Check sheet for the drawn part. Datum: minimum x, y, z corner. Units: mm. A direction names the side the tool comes from. Coordinates: 2 decimals unless noted, no trailing zeros. Write each loop counter-clockwise with the first axis right and the second up, starting at its lowest first coordinate (ties: lowest second). Pieces come first, ordered by that corner, then holes. Notation, with made-up numbers: (-10.5, 33.5) -> (37.5, 33.5) arc R37 ccw to (37.5, 72.5) -> close; hole circle Ø5 at (84, -33.5). An arc over 180 degrees is marked (long way). Answer in a Markdown table with one row per item. Add a question column.
1. Depth check by flat-ended pin: P1, Ø4, axis at x = 11.5, y = 16.5, coming from the -Z side; P2, Ø12, axis at x = 14, z = 17.5, coming from the -Y side; P3, Ø1.6, axis at x = 11.5, y = 17.5, coming from the -Z side. Enter the tip coordinate at first touch or a pass-through.
2. Set-up check for the marked faces 1 and 2: record each of +Z, -Z, +X, -X, +Y, -Y from which the full face is reachable in a straight line by a thin tool's end or side.
3. Mould release check, pull along X, two halves, no side actions. Record for the marked faces 3 and 4: pulls with the +X half, pulls with the -X half, needs draft (parallel to the pull), parting line crosses it, or undercut.
4. Cross-section at C-C on z = 10.5. Record the cut outline in (x, y), and give its area (3 significant figures).
5. Cross-section at B-B on z = 17.5. Record the cut outline in (x, y), and give its area (3 significant figures).
6. Cross-section at A-A on x = 11.4. Record the cut outline in (y, z), and give its area (3 significant figures).
7. Scan lines: L1, parallel to Z at x = 7, y = 11.75; L2, parallel to Y at x = 17.25, z = 2.75; L3, parallel to Y at x = 5.4, z = 3.15. Record each from-to range of solid material in increasing order. Write a range as from..to.
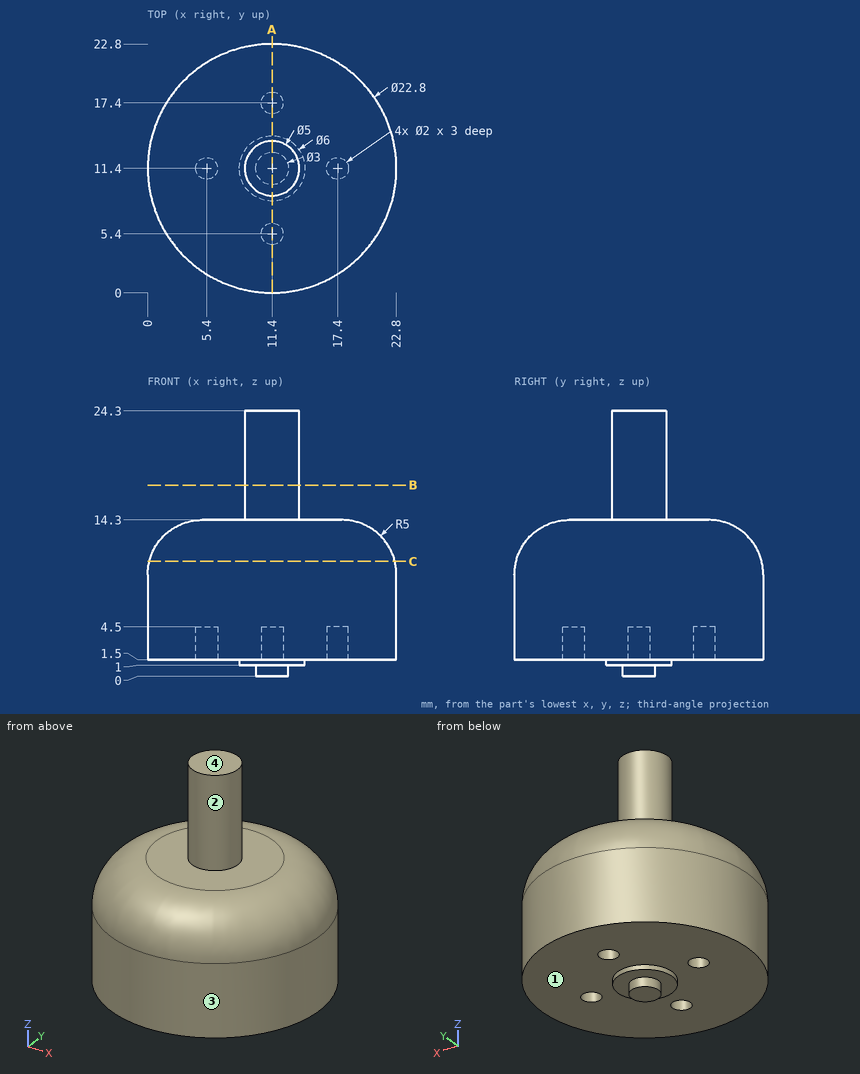
Results found:
| question | item | result |
|---|---|---|
| 1 | P1 | stops at z = 1.5 |
| 1 | P2 | stops at y = 0.66 |
| 1 | P3 | stops at z = 4.5 |
| 2 | face 1 | -Z |
| 2 | face 2 | +Z |
| 3 | face 3 | parting line crosses it |
| 3 | face 4 | needs draft |
| 4 | outline | circle Ø22.51 at (11.4, 11.4) |
| 4 | area | 398 mm^2 |
| 5 | outline | circle Ø5 at (11.4, 11.4) |
| 5 | area | 19.6 mm^2 |
| 6 | outline | (0, 1.5) -> (4.4, 1.5) -> (4.4, 4.5) -> (6.4, 4.5) -> (6.4, 1.5) -> (8.4, 1.5) -> (8.4, 1) -> (9.9, 1) -> (9.9, 0) -> (12.9, 0) -> (12.9, 1) -> (14.4, 1) -> (14.4, 1.5) -> (16.4, 1.5) -> (16.4, 4.5) -> (18.4, 4.5) -> (18.4, 1.5) -> (22.8, 1.5) -> (22.8, 9.3) arc R5 ccw to (17.8, 14.3) -> (13.9, 14.3) -> (13.9, 24.3) -> (8.9, 24.3) -> (8.9, 14.3) -> (5, 14.3) arc R5 ccw to (0, 9.3) -> close |
| 6 | area | 325 mm^2 |
| 7 | L1 | z = 1.5..14.3 |
| 7 | L2 | y = 1.62..10.41, 12.39..21.18 |
| 7 | L3 | y = 1.71..10.4, 12.4..21.09 |
